from build123d import *

# Parameters (mm, degrees)
F0_W          = 127
F0_H          = 152.4
F1_DEPTH      = 12.7
F2_T          = -5.08
F3_R          = 6.35
F4_DEPTH      = 101.6
F4_DEPTH_BACK = 7.62
F5_R          = 10.16
F6_T1_DEPTH   = 132.08
F6_T3_DEPTH   = 106.68
F6_T6_ANGLE   = 90
F6_T8_ANGLE   = 90
F6_T10_ANGLE  = 90
F6_T12_ANGLE  = 90
F6_T14_ANGLE  = 90
F6_T16_ANGLE  = 90
F6_T18_ANGLE  = 90
F6_T20_ANGLE  = 90
F7_SIZE       = 2.54


# Not quite as in the source:
# - a fillet or chamfer that OpenCascade refuses, or shapes differently, is made with other operations: its cross-section is extruded or revolved along the edge and cut away or added


with BuildPart() as f1:
    # F0 (on Top) → F1 (new body)
    with BuildSketch(Plane.XY):
        Rectangle(F0_W, F0_H)
    extrude(amount=-F1_DEPTH)

    # F2
    f2_openings = [f1.faces().sort_by_distance(p)[0] for p in [
        (0, 0, -12.7),
    ]]
    offset(amount=F2_T, openings=f2_openings)

    # F3 (on face) → F4 (join, two sides)
    with BuildSketch(Plane(origin=(0, 0, -12.7), x_dir=(1, 0, 0), z_dir=(0, 0, -1))) as f4_sk:
        with Locations((-50.8, 63.5)):
            Circle(F3_R)
        with Locations((50.8, 63.5)):
            Circle(F3_R)
        with Locations((50.8, -63.5)):
            Circle(F3_R)
        with Locations((-50.8, -63.5)):
            Circle(F3_R)
    extrude(amount=F4_DEPTH)
    extrude(f4_sk.sketch, amount=-F4_DEPTH_BACK)

    # F5
    f5_edges = [f1.edges().sort_by_distance(p)[0] for p in [
        (-63.5, -76.2, -6.35),
        (-63.5, 76.2, -6.35),
        (63.5, 76.2, -6.35),
        (63.5, -76.2, -6.35),
    ]]
    fillet(f5_edges, radius=F5_R)

    # F6: fillet of radius 5.08 on 18 edges, made by hand

    # F6_s2 → F6_t1 (cut)
    with BuildSketch(Plane.XZ.offset(-66.04)):
        with BuildLine():
            ThreePointArc((-58.42, 0), (-62.0121024484, -1.4878975516), (-63.5, -5.08))
            Line((-63.5, -5.08), (-63.5, 0))
            Line((-63.5, 0), (-58.42, 0))
        make_face()
        with BuildLine():
            ThreePointArc((-58.42, -12.7), (-62.0121024484, -11.2121024484), (-63.5, -7.62))
            Line((-63.5, -7.62), (-63.5, -12.7))
            Line((-63.5, -12.7), (-58.42, -12.7))
        make_face()
        with BuildLine():
            ThreePointArc((58.42, 0), (62.0121024484, -1.4878975516), (63.5, -5.08))
            Line((63.5, -5.08), (63.5, 0))
            Line((63.5, 0), (58.42, 0))
        make_face()
        with BuildLine():
            ThreePointArc((58.42, -12.7), (62.0121024484, -11.2121024484), (63.5, -7.62))
            Line((63.5, -7.62), (63.5, -12.7))
            Line((63.5, -12.7), (58.42, -12.7))
        make_face()
    extrude(amount=F6_T1_DEPTH, mode=Mode.SUBTRACT)

    # F6_s4 → F6_t3 (cut)
    with BuildSketch(Plane.YZ.offset(-53.34)):
        with BuildLine():
            ThreePointArc((-76.2, -5.08), (-74.7121024484, -1.4878975516), (-71.12, 0))
            Line((-71.12, 0), (-76.2, 0))
            Line((-76.2, 0), (-76.2, -5.08))
        make_face()
        with BuildLine():
            ThreePointArc((-76.2, -7.62), (-74.7121024484, -11.2121024484), (-71.12, -12.7))
            Line((-71.12, -12.7), (-76.2, -12.7))
            Line((-76.2, -12.7), (-76.2, -7.62))
        make_face()
        with BuildLine():
            ThreePointArc((71.12, 0), (74.7121024484, -1.4878975516), (76.2, -5.08))
            Line((76.2, -5.08), (76.2, 0))
            Line((76.2, 0), (71.12, 0))
        make_face()
        with BuildLine():
            ThreePointArc((71.12, -12.7), (74.7121024484, -11.2121024484), (76.2, -7.62))
            Line((76.2, -7.62), (76.2, -12.7))
            Line((76.2, -12.7), (71.12, -12.7))
        make_face()
    extrude(amount=F6_T3_DEPTH, mode=Mode.SUBTRACT)

    # F6_s5 → F6_t6 (revolve, cut)
    with BuildSketch(Plane.YZ.offset(-53.34)):
        with BuildLine():
            ThreePointArc((-71.12, 0), (-74.7121024484, -1.4878975516), (-76.2, -5.08))
            Line((-76.2, -5.08), (-76.2, 0))
            Line((-76.2, 0), (-71.12, 0))
        make_face()
    revolve(axis=Axis((-53.34, -66.04, 0), (0, 0, -1)), revolution_arc=F6_T6_ANGLE, mode=Mode.SUBTRACT)

    # F6_s7 → F6_t8 (revolve, cut)
    with BuildSketch(Plane.YZ.offset(53.34)):
        with BuildLine():
            ThreePointArc((-71.12, 0), (-74.7121024484, -1.4878975516), (-76.2, -5.08))
            Line((-76.2, -5.08), (-76.2, 0))
            Line((-76.2, 0), (-71.12, 0))
        make_face()
    revolve(axis=Axis((53.34, -66.04, 0), (0, 0, 1)), revolution_arc=F6_T8_ANGLE, mode=Mode.SUBTRACT)

    # F6_s9 → F6_t10 (revolve, cut)
    with BuildSketch(Plane.YZ.offset(-53.34)):
        with BuildLine():
            ThreePointArc((71.12, 0), (74.7121024484, -1.4878975516), (76.2, -5.08))
            Line((76.2, -5.08), (76.2, 0))
            Line((76.2, 0), (71.12, 0))
        make_face()
    revolve(axis=Axis((-53.34, 66.04, 0), (0, 0, 1)), revolution_arc=F6_T10_ANGLE, mode=Mode.SUBTRACT)

    # F6_s11 → F6_t12 (revolve, cut)
    with BuildSketch(Plane.YZ.offset(53.34)):
        with BuildLine():
            ThreePointArc((71.12, 0), (74.7121024484, -1.4878975516), (76.2, -5.08))
            Line((76.2, -5.08), (76.2, 0))
            Line((76.2, 0), (71.12, 0))
        make_face()
    revolve(axis=Axis((53.34, 66.04, 0), (0, 0, -1)), revolution_arc=F6_T12_ANGLE, mode=Mode.SUBTRACT)

    # F6_s13 → F6_t14 (revolve, cut)
    with BuildSketch(Plane.YZ.offset(-53.34)):
        with BuildLine():
            ThreePointArc((-76.2, -7.62), (-74.7121024484, -11.2121024484), (-71.12, -12.7))
            Line((-71.12, -12.7), (-76.2, -12.7))
            Line((-76.2, -12.7), (-76.2, -7.62))
        make_face()
    revolve(axis=Axis((-53.34, -66.04, -12.7), (0, 0, -1)), revolution_arc=F6_T14_ANGLE, mode=Mode.SUBTRACT)

    # F6_s15 → F6_t16 (revolve, cut)
    with BuildSketch(Plane.YZ.offset(53.34)):
        with BuildLine():
            ThreePointArc((-76.2, -7.62), (-74.7121024484, -11.2121024484), (-71.12, -12.7))
            Line((-71.12, -12.7), (-76.2, -12.7))
            Line((-76.2, -12.7), (-76.2, -7.62))
        make_face()
    revolve(axis=Axis((53.34, -66.04, -12.7), (0, 0, 1)), revolution_arc=F6_T16_ANGLE, mode=Mode.SUBTRACT)

    # F6_s17 → F6_t18 (revolve, cut)
    with BuildSketch(Plane.YZ.offset(-53.34)):
        with BuildLine():
            ThreePointArc((71.12, -12.7), (74.7121024484, -11.2121024484), (76.2, -7.62))
            Line((76.2, -7.62), (76.2, -12.7))
            Line((76.2, -12.7), (71.12, -12.7))
        make_face()
    revolve(axis=Axis((-53.34, 66.04, -12.7), (0, 0, 1)), revolution_arc=F6_T18_ANGLE, mode=Mode.SUBTRACT)

    # F6_s19 → F6_t20 (revolve, cut)
    with BuildSketch(Plane.YZ.offset(53.34)):
        with BuildLine():
            ThreePointArc((71.12, -12.7), (74.7121024484, -11.2121024484), (76.2, -7.62))
            Line((76.2, -7.62), (76.2, -12.7))
            Line((76.2, -12.7), (71.12, -12.7))
        make_face()
    revolve(axis=Axis((53.34, 66.04, -12.7), (0, 0, -1)), revolution_arc=F6_T20_ANGLE, mode=Mode.SUBTRACT)

    # F7
    f7_edges = [f1.edges().sort_by_distance(p)[0] for p in [
        (-57.15, -63.5, -114.3),
        (44.45, -63.5, -114.3),
        (-57.15, 63.5, -114.3),
        (44.45, 63.5, -114.3),
    ]]
    chamfer(f7_edges, length=F7_SIZE)


solid = f1.part
The listing builds one solid part. Answer for the finished solid, in the listing's coordinates (mm). A direction names the side the tool comes from. Give positions to 0.01 mm unless a question says otherwise; leave off trailing zeros. Write each loop counter-clockwise with the first axis right and the second up, starting at its lowest first coordinate (ties: lowest second). Pieces come first, ordered by that corner, then holes. Notation, with made-up numbers: (-13, 63) -> (39, 63) arc R30 ccw to (39, 98) -> close; hole circle Ø11 at (-25, 9.5). An arc over 180 degrees is marked (long way). One line per question, with ' | ' between items. Start each with the question number.
1. Section B-B (x = -2) is taken. Determine the outline of the cut face in (y, z), plus the area to 3 significant figures.
2. Section D-D (x = 50.8) is taken. Determine the outline of the cut face in (y, z).
3. Find the intervals of material crossed by probe 1 along Y at (x, z) = (51.5, -53); probe 2 along Z at (x, y) = (4, -56.5); probe 3 along Y at (x, z) = (49, -70.5), in increasing order.
4. Section A-A (y = 63.5) is taken. Determine the outline of the cut face in (x, z), plus the area to 3 significant figures.
5. For faces 1 (the flat face through (-1, 1, -5.08)), 2 (the cylindrical face through (-60.445, 73.303, -6.368)), determine the directions among +Z, -Z, +X, -X, +Y, -Y from which every point of the face is accessible in a straight line to the end or side of a thin tool.
6. Section C-C (z = -54) is taken. Determine the outline of the cut face in (x, y), plus the area to 3 significant figures.
7. Given pin 1 Ø3 at (x, y) = (48, 7) entering from -Z; pin 2 Ø10 at (y, z) = (47.5, -17) entering from -X; pin 3 Ø2.5 at (x, z) = (2.5, -10) entering from +Y, each flat-ended and moving along its own axis, determine where each tip first touches the part or whether it passes through.
8. For a pull along X with two mould halves and no side action, classify faces 3 (the flat face through (-1, 71.12, -9)), 4 (the flat face through (-1, 1, 0)), 5 (the cylindrical face through (-60.445, -73.303, -6.368)) as pulls with the +X half, pulls with the -X half, needs draft (parallel to the pull), parting line crosses it, or undercut.
Response values:
1) outline: (-76.2, -7.62) arc R5.08 ccw to (-71.12, -12.7) -> (-71.12, -5.08) -> (71.12, -5.08) -> (71.12, -12.7) arc R5.08 ccw to (76.2, -7.62) -> (76.2, -5.08) arc R5.08 ccw to (71.12, 0) -> (-71.12, 0) arc R5.08 ccw to (-76.2, -5.08) -> close | area: 829 mm2
2) outline: (-76.2, -7.62) arc R5.08 ccw to (-71.12, -12.7) -> (-71.12, -5.08) -> (-69.85, -5.08) -> (-69.85, -111.76) -> (-67.31, -114.3) -> (-59.69, -114.3) -> (-57.15, -111.76) -> (-57.15, -5.08) -> (57.15, -5.08) -> (57.15, -111.76) -> (59.69, -114.3) -> (67.31, -114.3) -> (69.85, -111.76) -> (69.85, -5.08) -> (71.12, -5.08) -> (71.12, -12.7) arc R5.08 ccw to (76.2, -7.62) -> (76.2, -5.08) arc R5.08 ccw to (71.12, 0) -> (-71.12, 0) arc R5.08 ccw to (-76.2, -5.08) -> close
3) probe 1: -69.81 to -57.19, 57.19 to 69.81 | probe 2: -5.08 to 0 | probe 3: -69.59 to -57.41, 57.41 to 69.59
4) outline: (-63.5, -7.62) arc R5.08 ccw to (-58.42, -12.7) -> (-58.42, -5.08) -> (-57.15, -5.08) -> (-57.15, -111.76) -> (-54.61, -114.3) -> (-46.99, -114.3) -> (-44.45, -111.76) -> (-44.45, -5.08) -> (44.45, -5.08) -> (44.45, -111.76) -> (46.99, -114.3) -> (54.61, -114.3) -> (57.15, -111.76) -> (57.15, -5.08) -> (58.42, -5.08) -> (58.42, -12.7) arc R5.08 ccw to (63.5, -7.62) -> (63.5, -5.08) arc R5.08 ccw to (58.42, 0) -> (-58.42, 0) arc R5.08 ccw to (-63.5, -5.08) -> close | area: 3,460 mm2
5) face 1: -Z | face 2: +Z, -Z, -X, +Y
6) outline: circle Ø12.7 at (-50.8, -63.5); circle Ø12.7 at (-50.8, 63.5); circle Ø12.7 at (50.8, -63.5); circle Ø12.7 at (50.8, 63.5) | area: 507 mm2
7) pin 1: z = -5.08 | pin 2: x = -60.99 | pin 3: y = 76.07
8) face 3: undercut | face 4: needs draft | face 5: pulls with the -X half
